Geometry: final body of the model. Coordinates: model frame, mm. Face numbers are marked on the shaded views. A direction names the side the tool comes from. Round coordinates to 2 decimals unless told otherwise and drop trailing zeros. Write each loop counter-clockwise with the first axis right and the second up, starting at its lowest first coordinate (ties: lowest second). Pieces come first, ordered by that corner, then holes. Notation, with made-up numbers: (46, 17) - (65, 17) arc R18 cw to (65, 48) - close; hole circle Ø1 at (30.25, 59.25). An arc over 180 degrees is marked (long way). Write each question's results on one line, items separated by ' | '.
Autodesk Inventor part; units mm, degrees
ref_plane "YZ Plane" through (0, 0, 0) normal (1, 0, 0) x (0, 1, 0)
ref_plane "XZ Plane" through (0, 0, 0) normal (0, 1, 0) x (-1, 0, 0)
ref_plane "XY Plane" through (0, 0, 0) normal (0, 0, 1) x (1, 0, 0)
sketch "スケッチ1" plane through (0, 0, 0) normal (0, 0, 1) x (1, 0, 0)
  line L0 (-26.75, 0) -> (26.75, 0)
  line L1 (26.75, 0) -> (26.75, -26)
  line L2 (5, -24) -> (5, -7)
  line L3 (5, -7) -> (-5, -7)
  line L4 (-5, -7) -> (-5, -24)
  line L5 (-26.75, -26) -> (-26.75, 0)
  line L6 (-26.75, -26) -> (-20, -26)
  line L7 (-20, -26) -> (-20, -24)
  line L8 (-20, -24) -> (-5, -24)
  line L9 (5, -24) -> (20, -24)
  line L10 (20, -24) -> (20, -26)
  line L11 (20, -26) -> (26.75, -26)
  point P0 (0, 0)
  dimension "d0" = 53.5
  dimension "d1" = 10
  dimension "d2" = 5
  dimension "d3" = 26.75
  dimension "d4" = 40
  dimension "d5" = 20
  dimension "d6" = 17
  dimension "d7" = 2
  dimension "d29" = 24
extrude "押し出し1" add sketch "スケッチ1" along normal mid plane 15
sketch "スケッチ2" plane through (-26.75, 0, 7.5) normal (0, 1, 0) x (1, 0, 0)
  point P0 (26.75, 7.5)
  point P1 (16.75, 7.5)
  point P2 (36.75, 7.5)
  dimension "d11" = 10
  dimension "d12" = 10
hole "穴1" at (-10, 0, 0) at (10, 0, 0) direction (0, -1, 0) diameter 5.5 end through all counterbore diameter 9 counterbore depth 8
sketch "スケッチ3" plane through (-26.75, 0, 7.5) normal (0, 1, 0) x (1, 0, 0)
  point P0 (26.75, 7.5)
  point P1 (5, 7.5)
  point P2 (48.5, 7.5)
  dimension "d20" = 21.75
  dimension "d21" = 21.75
hole "穴2" at (-21.75, 0, 0) at (21.75, 0, 0) direction (0, -1, 0) diameter 5 depth 6 tip angle 118
fillet "フィレット1" radius 2 4 edges at (-26.75, -13, -7.5) (-26.75, -13, 7.5) (26.75, -13, -7.5) (26.75, -13, 7.5)
fillet "フィレット2" radius 2 2 edges at (5, -7, 0) (-5, -7, 0)
properties part number "scara-base7" material "ABS プラスチック"
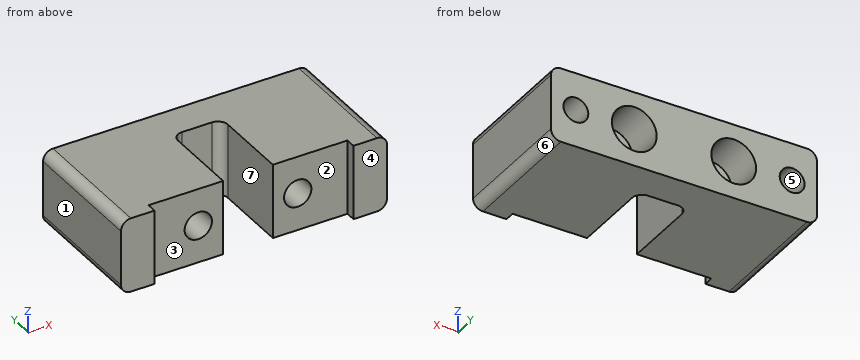
Q1. Section query B-B, the plane x = -10. Return loops of the section in (y, z), plus the area to 3 significant figures.
Answer block:
outline: (-24, -7.5) - (0, -7.5) - (0, -4.5) - (-8, -4.5) - (-8, -2.75) - (-24, -2.75) - close; (-24, 2.75) - (-8, 2.75) - (-8, 4.5) - (0, 4.5) - (0, 7.5) - (-24, 7.5) - close | area: 200 mm2
Q2. Section query A-A, the plane y = -15.25. Return loops of the section in (x, z).
Answer block:
outline: (-26.75, -5.5) arc R2 ccw to (-24.75, -7.5) - (-5, -7.5) - (-5, 7.5) - (-24.75, 7.5) arc R2 ccw to (-26.75, 5.5) - close; (5, -7.5) - (24.75, -7.5) arc R2 ccw to (26.75, -5.5) - (26.75, 5.5) arc R2 ccw to (24.75, 7.5) - (5, 7.5) - close; hole circle Ø5.5 at (-10, 0); hole circle Ø5.5 at (10, 0)
Q3. Pin query (flat end, axial travel): pin 1 (6.5 mm diameter, centred on x = -1, z = -3.5, fed in from -Y); pin 2 (1 mm diameter, centred on x = 13.5, z = -0.5, fed in from +Y); pin 3 (7.5 mm diameter, centred on x = 16, z = 3, fed in from -Y). Return the tip coordinate at first contact, or that it passes through.
Answer block:
pin 1: y = -7.44 | pin 2: y = -8 | pin 3: y = -24
Q4. Mould query, pull axis X, two halves, no side actions, for the marked faces 1, 2, 3 and 4. Classes: pulls with the +X half, pulls with the -X half, needs draft (parallel to the pull), parting line crosses it, or undercut.
Answer block:
face 1: pulls with the -X half | face 2: undercut | face 3: undercut | face 4: needs draft
Q5. Section query D-D, the plane x = -1.5. Return loops of the section in (y, z), plus the area to 3 significant figures.
Answer block:
outline: (-7, -7.5) - (0, -7.5) - (0, 7.5) - (-7, 7.5) - close | area: 105 mm2
Q6. Ray query, line 1 along X through (y, z) = (-18.25, -0.25); line 2 along X through (y, z) = (-1.5, 0.25); line 3 along Z through (x, y) = (10, -3.5). Return the intervals inside material, ascending.
Answer block:
line 1: -26.75 to -12.74, -7.26 to -5, 5 to 7.26, 12.74 to 26.75 | line 2: -26.75 to -24.24, -19.26 to -14.49, -5.51 to 5.51, 14.49 to 19.26, 24.24 to 26.75 | line 3: -7.5 to -4.5, 4.5 to 7.5
Q7. Section query C-C, the plane z = 5. Return loops of the section in (x, y), plus the area to 3 significant figures.
Answer block:
outline: (-26.75, -26) - (-20, -26) - (-20, -24) - (-5, -24) - (-5, -9) arc R2 cw to (-3, -7) - (3, -7) arc R2 cw to (5, -9) - (5, -24) - (20, -24) - (20, -26) - (26.75, -26) - (26.75, 0) - (-26.75, 0) - close | area: 1,140 mm2
Q8. Access query for the marked faces 5, 6 and 7. Directions: +Z, -Z, +X, -X, +Y, -Y. A direction counts if a zero-diameter tool reaches every point of the face in a straight line with its end or side. Return the directions, or none.
Answer block:
face 5: +Y | face 6: -Z, +X, +Y, -Y | face 7: +Z, -Z, -Y
